Part model, mm, in its own coordinate system. A direction names the side the tool comes from. Give positions to 0.01 mm unless a question says otherwise; leave off trailing zeros. Order: outer loops, then holes, each group sorted by start corner. A loop starts at its lowest first (then second) coordinate and runs counter-clockwise, first axis right, second up. Notation, with made-up numbers: M 70.5,22.25 L 107.5,22.25 A18 ccw 107.5,44.25 Z; hole C -23,64 d1. An arc over 180 degrees is marked long. Answer as a JSON object with one key per item and string values.
from build123d import *

# Parameters (mm, degrees)
F1_DEPTH = 70
F2_R     = 9
F3_DEPTH = 140.001


with BuildPart() as f1:
    # F0 (on Top) → F1 (new body)
    with BuildSketch(Plane.XY):
        with BuildLine():
            Line((-56, -70), (56, -70))
            ThreePointArc((56, -70), (65.899495, -65.899495), (70, -56))
            Line((70, -56), (70, 56))
            ThreePointArc((70, 56), (65.899495, 65.899495), (56, 70))
            Line((56, 70), (-56, 70))
            ThreePointArc((-56, 70), (-65.899495, 65.899495), (-70, 56))
            Line((-70, 56), (-70, -56))
            ThreePointArc((-70, -56), (-65.899495, -65.899495), (-56, -70))
        make_face()
        with BuildLine():
            ThreePointArc((-56, -65), (-62.363961, -62.363961), (-65, -56))
            Line((-65, -56), (-65, 56))
            ThreePointArc((-65, 56), (-62.363961, 62.363961), (-56, 65))
            Line((-56, 65), (56, 65))
            ThreePointArc((56, 65), (62.363961, 62.363961), (65, 56))
            Line((65, 56), (65, -56))
            ThreePointArc((65, -56), (62.363961, -62.363961), (56, -65))
            Line((56, -65), (-56, -65))
        make_face(mode=Mode.SUBTRACT)
    extrude(amount=F1_DEPTH)

    # F2 (on face) → F3 (cut, through all)
    with BuildSketch(Plane.YZ.offset(70)):
        with Locations((0, 40)):
            Circle(F2_R)
    extrude(amount=-F3_DEPTH, mode=Mode.SUBTRACT)


solid = f1.part
1. Cut at A-A on z = 40. Give the cut face in (x, y).
Worked answers:
{"outline": "M -70,-56 A14 ccw -56,-70 L 56,-70 A14 ccw 70,-56 L 70,-9 L 65,-9 L 65,-56 A9 cw 56,-65 L -56,-65 A9 cw -65,-56 L -65,-9 L -70,-9 Z; M -70,9 L -65,9 L -65,56 A9 cw -56,65 L 56,65 A9 cw 65,56 L 65,9 L 70,9 L 70,56 A14 ccw 56,70 L -56,70 A14 ccw -70,56 Z"}
2. Cut at B-B on x = -3.5. Give the cut face in (y, z), plus the area to 3 significant figures.
Worked answers:
{"outline": "M -70,0 L -65,0 L -65,70 L -70,70 Z; M 65,0 L 70,0 L 70,70 L 65,70 Z", "area": "700 mm^2"}
3. Two-plate mould, pull along X, no slides. Class faces 1 (the cylindrical face through (65.8, -66, 34.5)), 2 (the cylindrical face through (62.294, 62.434, 34.51)), 3 (the flat face through (-1, 65, 35)), 4 (the flat face through (-1, -70, 35)): +X half, -X half, draft (parallel to the pull), parting line (faces both ways), or undercut.
Worked answers:
{"face 1": "+X half", "face 2": "undercut", "face 3": "undercut", "face 4": "draft"}
4. Which spindle directions (+Z, -Z, +X, -X, +Y, -Y) get a long thin tool onto all of the face, cutting with end or side? Do faces 5 (the flat face through (65, 1, 27)), 6 (the cylindrical face through (-66, -65.8, 34.5)). Say none if no direction does.
Worked answers:
{"face 5": "+Z, -Z", "face 6": "+Z, -Z, -X, -Y"}
5. Probe line 1 along X through (y, z) = (-15.5, 46); line 2 along Z through (x, y) = (67, 0). List the from-to ranges inside material, lowest first.
Worked answers:
{"line 1": "x = -70 to -65, 65 to 70", "line 2": "z = 0 to 31, 49 to 70"}
6. Cut at D-D on y = 0. Give the cut face in (x, z).
Worked answers:
{"outline": "M -70,0 L -65,0 L -65,31 L -70,31 Z; M -70,49 L -65,49 L -65,70 L -70,70 Z; M 65,0 L 70,0 L 70,31 L 65,31 Z; M 65,49 L 70,49 L 70,70 L 65,70 Z"}
